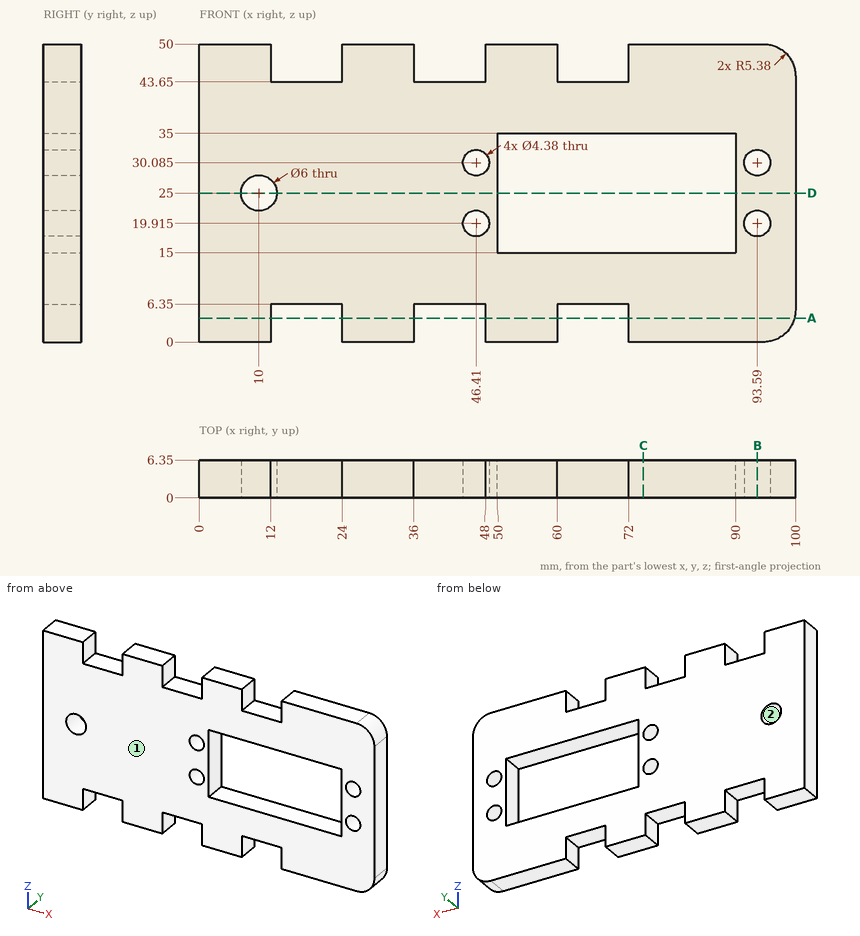
For this review, use the dimensioned drawing (mm, ordinates from the lowest corner) and the shaded views. Coordinates: 2 decimals unless noted, no trailing zeros. Loops run counter-clockwise (first coordinate to the right, second up) from the corner with the lowest first, then second, coordinate; pieces in that order, holes last.
1. Add section B-B, the plane x = 93.59. Give the boundary of the cut face in (y, z) (3 decimals), then the cut area to 3 significant figures.
2. Add section C-C, the plane x = 74.5. Give the boundary of the cut face in (y, z), then the cut area to 4 significant figures.
3. Add section A-A, the plane z = 4. Give the boundary of the cut face in (x, y), then the cut area to 3 significant figures.
4. Add section D-D, the plane z = 25. Give the boundary of the cut face in (x, y).
5. Mouldability with a two-part tool opening along X and no side actions: class the marked faces 1 and 2 as +X half, -X half, draft (parallel to the pull), parting line (faces both ways), or undercut.
6. For line 1 (X direction, y = 2, z = 25); line 2 (Z direction, x = 75.5, y = 2.25); line 3 (X direction, y = 3, z = 26), list the stretches that pass through material, from the lowest coordinate up.
7. Insertion check: P1, Ø1.9, axis at x = 20.5, y = 3.5, coming from the +Z side; P2, Ø3, axis at x = 19.5, y = 1.5, coming from the -Z side; P3, Ø3, axis at y = 4.5, z = 48, coming from the +X side; P4, Ø5.5, axis at x = 10, z = 25, coming from the +Y side. Each pin has a flat end and moves straight along its axis. Give the tip position at first contact, or say it passes through.
Result:
1. outline: (0, 0) - (6.35, 0) - (6.35, 17.725) - (0, 17.725) - close; (0, 22.105) - (6.35, 22.105) - (6.35, 27.895) - (0, 27.895) - close; (0, 32.275) - (6.35, 32.275) - (6.35, 50) - (0, 50) - close
1. area: 262 mm2
2. outline: (0, 0) - (6.35, 0) - (6.35, 15) - (0, 15) - close; (0, 35) - (6.35, 35) - (6.35, 50) - (0, 50) - close
2. area: 190.5 mm2
3. outline: (0, 0) - (12, 0) - (12, 6.35) - (0, 6.35) - close; (24, 0) - (36, 0) - (36, 6.35) - (24, 6.35) - close; (48, 0) - (60, 0) - (60, 6.35) - (48, 6.35) - close; (72, 0) - (99.82, 0) - (99.82, 6.35) - (72, 6.35) - close
3. area: 405 mm2
4. outline: (0, 0) - (7, 0) - (7, 6.35) - (0, 6.35) - close; (13, 0) - (50, 0) - (50, 6.35) - (13, 6.35) - close; (90, 0) - (100, 0) - (100, 6.35) - (90, 6.35) - close
5. face 1: draft
5. face 2: undercut
6. line 1: x = 0 to 7, 13 to 50, 90 to 100
6. line 2: z = 0 to 15, 35 to 50
6. line 3: x = 0 to 7.17, 12.83 to 50, 90 to 100
7. P1: stops at z = 43.65
7. P2: stops at z = 6.35
7. P3: stops at x = 99.66
7. P4: passes through
